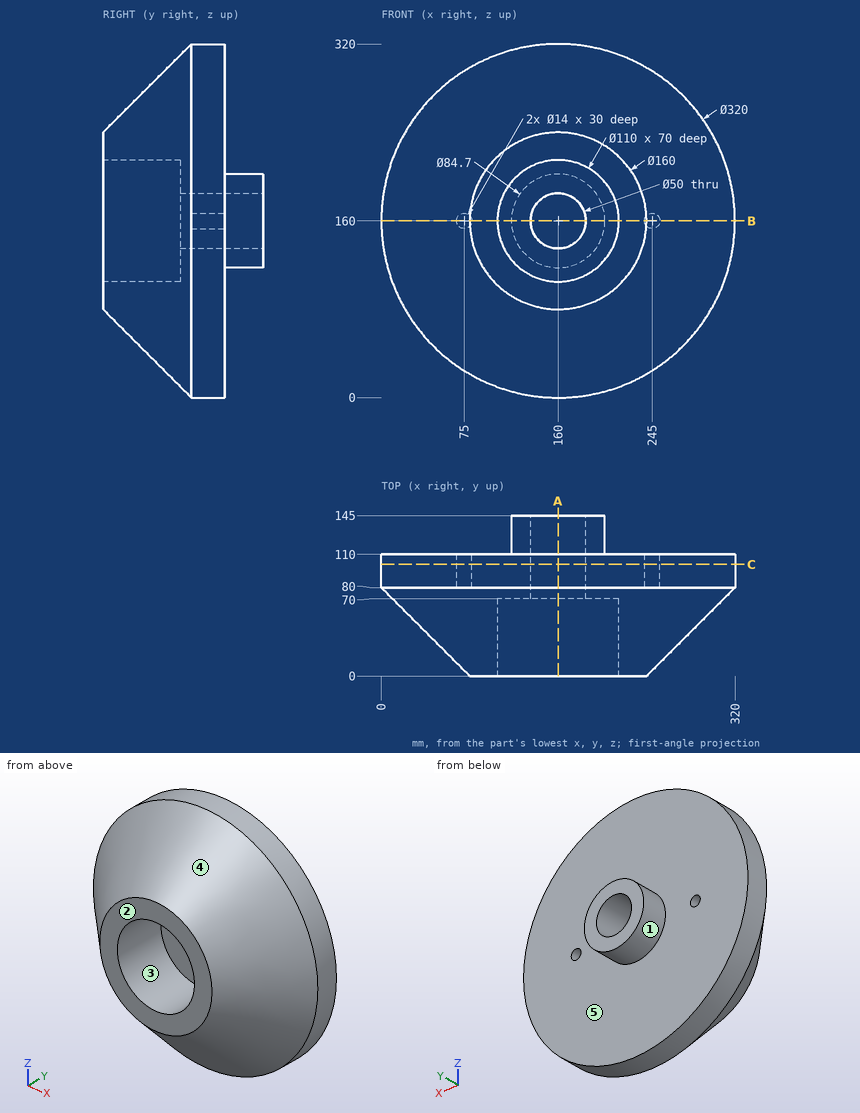
Design review of the part shown in the three views and the two pictorial views. Dimensions are in mm from the part's minimum x, y and z. A direction names the side the tool comes from. Give positions to 0.01 mm unless a question says otherwise; leave off trailing zeros. Write each loop counter-clockwise with the first axis right and the second up, starting at its lowest first coordinate (ties: lowest second). Pieces come first, ordered by that corner, then holes. Notation, with made-up numbers: M 6.5,79 L 63.5,79 A23 cw 63.5,103 Z; hole C -21.5,58 d10. An arc over 180 degrees is marked long. One line per question, with ' | ' between items. Start each with the question number.
Item 1: Draft analysis for pull direction X (two halves, no side actions). For the marked faces 1, 2 and 3, state which applies: released by +X, released by -X, zero draft, split by the parting line, or undercut.
Item 2: We need section B-B on z = 160. Write out the cut boundary in (x, y).
Item 3: Wall thickness on line 1 (Z direction, x = 160, y = 88.5); line 2 (Z direction, x = 75, y = 103.5); line 3 (X direction, y = 51, z = 122): over which ranges is each line inside the solid? List them lowest first. Write a range as from..to.
Item 4: We need section C-C on y = 101. Write out the cut boundary in (x, z).
Item 5: For the marked faces 4 and 5, list the 3-axis set-ups (+Z, -Z, +X, -X, +Y, -Y) from which the entire face can be reached by the end or side of a thin tool; tool diameter is ignored.
Item 6: We need section A-A on x = 160. Write out the cut boundary in (y, z).
Item 7: For pin 1 (2 mm diameter, centred on x = 181.5, z = 224, fed in from +Y); pin 2 (12 mm diameter, centred on y = 23.5, z = 104, fed in from +X); pin 3 (4 mm diameter, centred on x = 58, z = 40.5, fed in from -Y); pin 4 (16 mm diameter, centred on x = 245, z = 160, fed in from -Y), all flat-tipped, find the tip position at first contact; note any pin that passes through.
Results found:
1) face 1: split by the parting line | face 2: zero draft | face 3: undercut
2) outline: M 0,80 L 80,0 L 105,0 L 105,70 L 135,70 L 135,145 L 117.65,145 L 117.65,110 L 82,110 L 82,80 L 68,80 L 68,110 L 0,110 Z; M 185,70 L 215,70 L 215,0 L 240,0 L 320,80 L 320,110 L 252,110 L 252,80 L 238,80 L 238,110 L 202.35,110 L 202.35,145 L 185,145 Z
3) line 1: z = 0..135, 185..320 | line 2: z = 24.45..153, 167..295.55 | line 3: x = 34.63..120.24, 199.76..285.37
4) outline: C 160,160 d320; hole C 75,160 d14; hole C 160,160 d50; hole C 245,160 d14
5) face 4: -Y | face 5: +Y
6) outline: M 0,80 L 80,0 L 110,0 L 110,117.65 L 145,117.65 L 145,135 L 70,135 L 70,105 L 0,105 Z; M 0,215 L 70,215 L 70,185 L 145,185 L 145,202.35 L 110,202.35 L 110,320 L 80,320 L 0,240 Z
7) pin 1: stops at y = 110 | pin 2: stops at x = 254.92 | pin 3: stops at y = 75.11 | pin 4: stops at y = 0
